Check sheet for the modelled part. Datum: model origin and axes. Units: mm. Give positions to 0.01 mm unless a question says otherwise; leave off trailing zeros. Order: outer loops, then holes, each group sorted by start corner. A loop starts at its lowest first (then second) coordinate and runs counter-clockwise, first axis right, second up.
Item 1: Sectioned sample at A-A on y = 59.5. Record the boundary of the cut face in (x, z) (3 decimals).
Item 2: Material ranges on line 1 along X through (y, z) = (58, -2); line 2 along Y through (x, z) = (-4, -2.3); line 3 along Z through (x, y) = (-2, 22) (3 decimals), recorded low to high.
Item 3: Release check for a two-part mould opening along Y. For faces 1 (the flat face through (-1, -15.399, -2)), 2 (the flat face through (-1, 105.395, -2)), 3 (the flat face through (8, 45, -1.575)), 4 (the flat face through (-17, 46, 0)) record: released by +Y, released by -Y, zero draft, split by the parting line, or undercut.
from build123d import *

# Parameters (mm, degrees)
F1_W     = 74.2999784
F1_H     = 120.793891
F2_DEPTH = 3.175
F3_DEPTH = 1.5748
F5_DEPTH = 1.6012
F7_DEPTH = 187


# Not quite as in the source:
# - an extrude ends at something that could not be found from the text; its depth is read off the source's solid


with BuildPart() as f2:
    # F1 (on Top) → F2 (new body)
    with BuildSketch(Plane.XY):
        with Locations((0, 44.9976621)):
            Rectangle(F1_W, F1_H)
    extrude(amount=-F2_DEPTH)

    # F0 (on Top) → F3 (cut)
    with BuildSketch(Plane.XY):
        Polygon((-11.67892, 70.7573642), (-11.7499892, 70.4366892), (-10.0000054, 14.202029), (-9.1080082, 13.367766), (-8.146669, 12.614402), (-7.1233538, 11.9477028), (-6.045835, 11.372723), (-4.9222914, 10.8938568), (-3.7612828, 10.514711), (-2.5716484, 10.2382066), (-1.3624306, 10.0664518), (-0.142875, 10.0007166), (1.0777982, 10.0415598), (2.2902418, 10.1886004), (3.4852864, 10.4407716), (4.653788, 10.7961176), (5.7868566, 11.2519714), (6.875907, 11.8048532), (7.9126334, 12.4505212), (8.889111, 13.1840986), (9.7979484, 13.9999974), (10.0000054, 14.202029), (11.7499892, 70.4366892), (11.4929158, 71.4514954), (11.1483648, 72.440038), (10.7189524, 73.3947986), (10.2079806, 74.3084874), (9.6193102, 75.1741702), (8.957437, 75.985243), (8.2274156, 76.735559), (7.4347324, 77.4193778), (6.5855088, 78.0315178), (5.6861456, 78.5673054), (4.7435008, 79.0226766), (3.7647626, 79.3941516), (2.7573732, 79.678911), (1.728978, 79.8747958), (0.687451, 79.980282), (-0.3593084, 79.9946076), (-1.40335, 79.917671), (-2.4366982, 79.7500056), (-3.4515044, 79.4929068), (-4.440047, 79.1483558), (-5.3947822, 78.7189688), (-6.3084964, 78.207997), (-7.1741538, 77.6193266), (-7.985252, 76.9574534), (-8.7355426, 76.2274066), (-9.4193614, 75.4347488), (-10.0315014, 74.5854998), (-10.5673144, 73.6861366), (-11.0226602, 72.7434918), (-11.3941352, 71.7647536), align=None)
    extrude(amount=-F3_DEPTH, mode=Mode.SUBTRACT)

    # F4 (on face) → F5 (cut, through all)
    with BuildSketch(Plane.XY.offset(-1.5748)):
        Polygon((7.5, 74.9946076), (-7.5, 74.9946076), (-7.5, 29.9946076), (0, 29.9946076), (7.5, 29.9946076), align=None)
    extrude(amount=-F5_DEPTH, mode=Mode.SUBTRACT)

    # F6 (on Top) → F7 (cut, through all)
    with BuildSketch(Plane.XY):
        Polygon((-10.7912024307, 73.8066075367), (-11.2561967507, 72.8439886266), (-11.6355402146, 71.8445191089), (-11.9253249204, 70.8194431888), (-12.0048558585, 70.4605875443), (-10.2505992593, 14.0886235531), (-9.2734099156, 13.1746824405), (-8.2946132005, 12.4076376674), (-7.2527155028, 11.7288318004), (-6.155627842, 11.1434097699), (-5.0116809128, 10.6558474546), (-3.8295896081, 10.2698167625), (-2.6183487878, 9.9882904244), (-1.3871727116, 9.8134167162), (-0.1454684467, 9.7464876822), (1.0973724592, 9.7880726041), (2.3318323641, 9.9377832588), (3.5485785618, 10.1945338008), (4.7383012319, 10.5563332129), (5.8919487163, 11.0204662668), (7.0007735223, 11.5833870046), (8.0563268906, 12.240780346), (9.0505396482, 12.9876812578), (9.9727120125, 13.8155513756), (10.250752791, 14.0935572024), (12.00497648, 70.4644636422), (11.7364147609, 71.5246203819), (11.3845631065, 72.5341091055), (10.9460529906, 73.5090976745), (10.4242555991, 74.442144141), (9.8231127621, 75.3261685703), (9.1472184874, 76.1544230786), (8.4017288342, 76.9206373493), (7.5922505458, 77.6189446578), (6.7250358763, 78.2440530365), (5.8066165367, 78.7911931616), (4.8440002256, 79.2562121642), (3.8445253314, 79.6355576688), (2.8157931282, 79.9263500525), (1.7656080971, 80.1263852965), (0.7020137501, 80.2341064847), (-0.3669184196, 80.2487355339), (-1.4330803845, 80.1701688593), (-2.4883265282, 79.9989504193), (-3.5246322079, 79.7364047759), (-4.5341166426, 79.3845546164), (-5.509078548, 78.9460707649), (-6.4421534102, 78.4242719991), (-7.3261519012, 77.8231291621), (-8.154434062, 77.1472334884), (-8.9206223557, 76.4017179349), (-9.6189282578, 75.5922672148), (-10.2440360096, 74.725027477), align=None)
    extrude(amount=F7_DEPTH, mode=Mode.SUBTRACT)


solid = f2.part
Report:
1. outline: (-37.15, -3.175) - (-7.5, -3.175) - (-7.5, -1.575) - (-11.41, -1.575) - (-11.41, 0) - (-37.15, 0) - close; (7.5, -3.175) - (37.15, -3.175) - (37.15, 0) - (11.41, 0) - (11.41, -1.575) - (7.5, -1.575) - close
2. line 1: x = -37.15 to -7.5, 7.5 to 37.15
2. line 2: y = -15.4 to 29.99, 74.99 to 105.39
2. line 3: z = -3.175 to -1.575
3. face 1: released by -Y
3. face 2: released by +Y
3. face 3: undercut
3. face 4: zero draft
